Verification items for the finished model (mm, model axes). Face numbers are marked on the shaded views. A direction names the side the tool comes from. Give positions to 0.01 mm unless a question says otherwise; leave off trailing zeros. Loops run counter-clockwise (first coordinate to the right, second up) from the corner with the lowest first, then second, coordinate; pieces in that order, holes last. Notation, with made-up numbers: (51, 64.5) - (110, 64.5) arc R22 cw to (110, 80.5) - close; hole circle Ø2 at (-17.75, 2). An arc over 180 degrees is marked (long way). Answer in a Markdown table with one row per item.
Autodesk Fusion 360 part; units mm, degrees
sketch "Sketch2" plane through (0, 0, 0) normal (0, 0, 1) x (1, 0, 0)
  circle A0 centre (0, 0) radius 9
  circle A1 centre (0, 0) radius 8
  circle A2 centre (0, 0) radius 1.75
  dimension "d10" = 16
  dimension "d26" = 3.5
extrude "Extrude3" add sketch "Sketch2" along normal blind 5.2 contours A1
sketch "Sketch3" plane through (0, 0, 5.2) normal (0, 0, 1) x (1, 0, 0)
  circle A0 centre (0, 0) radius 6.05
  circle A1 centre (0, 0) radius 8
  circle A2 centre (0, 0) radius 1.75
  dimension "d13" = 12.1
extrude "Extrude4" add sketch "Sketch3" along normal blind 8 contours A0
sketch "Sketch4" plane through (0, 0, 13.2) normal (0, 0, 1) x (1, 0, 0)
  circle A0 centre (0, 0) radius 6.05
  line L0 (-1.963, 3.4) -> (-3.926, 0)
  line L1 (-3.926, 0) -> (-1.963, -3.4)
  line L2 (-1.963, -3.4) -> (1.963, -3.4)
  line L3 (1.963, -3.4) -> (3.926, 0)
  line L4 (3.926, 0) -> (1.963, 3.4)
  line L5 (1.963, 3.4) -> (-1.963, 3.4)
  circle A1 centre (0, 0) radius 1.75
  dimension "d24" = 6.8
extrude "Extrude5" add sketch "Sketch4" along normal blind 10 contours L0 L1 L2 L3 L4 L5
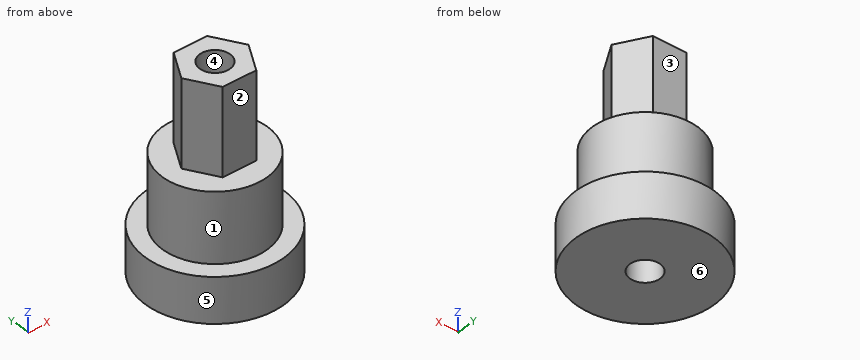
Q1. Sectioned sample at C-C (x = 3.5). Record the cut outline in (y, z), and give its area (3 significant figures).
Completed:
| item | result |
|---|---|
| outline | (-7.19, 0) - (7.19, 0) - (7.19, 5.2) - (4.93, 5.2) - (4.93, 13.2) - (0.74, 13.2) - (0.74, 23.2) - (-0.74, 23.2) - (-0.74, 13.2) - (-4.93, 13.2) - (-4.93, 5.2) - (-7.19, 5.2) - close |
| area | 169 mm^2 |
Q2. Sectioned sample at D-D (y = -2.5). Record the cut outline in (x, z), and give its area (3 significant figures).
Completed:
| item | result |
|---|---|
| outline | (-7.6, 0) - (7.6, 0) - (7.6, 5.2) - (5.51, 5.2) - (5.51, 13.2) - (2.48, 13.2) - (2.48, 23.2) - (-2.48, 23.2) - (-2.48, 13.2) - (-5.51, 13.2) - (-5.51, 5.2) - (-7.6, 5.2) - close |
| area | 217 mm^2 |
Q3. Thickness scan on line 1 (Y direction, x = 0, z = 12); line 2 (Z direction, x = 0, y = 3.5); line 3 (Z direction, x = 7.25, y = -0.25). Record the ranges inside material, lowest first.
Completed:
| item | result |
|---|---|
| line 1 | -6.05 to -1.75, 1.75 to 6.05 |
| line 2 | 0 to 13.2 |
| line 3 | 0 to 5.2 |
Q4. Go/stop test with flat-tipped pins: P1, Ø2, axis at x = 5, z = 11.5, coming from the +Y side; P2, Ø2, axis at x = -0.5, z = 19, coming from the -Y side; P3, Ø8, axis at x = 6, z = 6, coming from the -Y side. Record where each tip stops, or that it passes through.
Completed:
| item | result |
|---|---|
| P1 | y = 4.54 |
| P2 | y = -3.4 |
| P3 | y = -7.72 |
Q5. Tool access check on the marked faces 1, 2 and 3. Record the directions out of +Z, -Z, +X, -X, +Y, -Y that give a thin tool (end or side, any length) a straight path to the whole face; none if there is none.
Completed:
| item | result |
|---|---|
| face 1 | +Z |
| face 2 | +Z, +X, -X, -Y |
| face 3 | +Z, +X, -X, +Y |
Q6. Sectioned sample at B-B (z = 15). Record the cut outline in (x, y).
Completed:
| item | result |
|---|---|
| outline | (-3.93, 0) - (-1.96, -3.4) - (1.96, -3.4) - (3.93, 0) - (1.96, 3.4) - (-1.96, 3.4) - close; hole circle Ø3.5 at (0, 0) |
Q7. Draft check along Y on the marked faces 4, 5 and 6. Enter one of: +Y half, -Y half, draft (parallel to the pull), parting line (faces both ways), or undercut.
Completed:
| item | result |
|---|---|
| face 4 | undercut |
| face 5 | parting line |
| face 6 | draft |
Q8. Sectioned sample at A-A (x = 0). Record the cut outline in (y, z).
Completed:
| item | result |
|---|---|
| outline | (-8, 0) - (-1.75, 0) - (-1.75, 23.2) - (-3.4, 23.2) - (-3.4, 13.2) - (-6.05, 13.2) - (-6.05, 5.2) - (-8, 5.2) - close; (1.75, 0) - (8, 0) - (8, 5.2) - (6.05, 5.2) - (6.05, 13.2) - (3.4, 13.2) - (3.4, 23.2) - (1.75, 23.2) - close |
